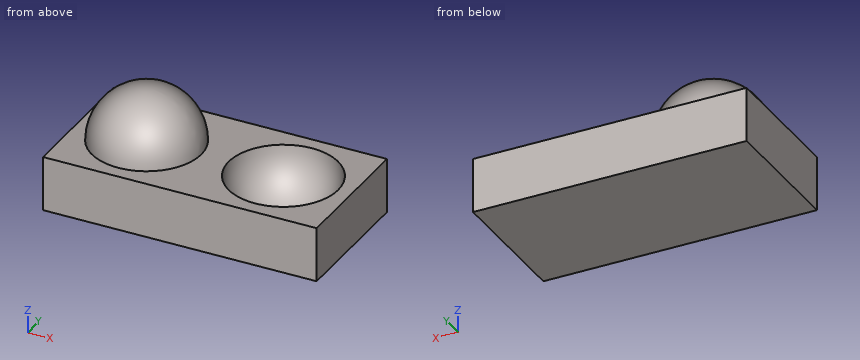
```python
from build123d import *

# Parameters (mm, degrees)
SKETCH_W  = 100
SKETCH_H  = 50
PAD_DEPTH = 20


with BuildPart() as part:
    # Sketch → Pad (new body)
    with BuildSketch(Plane.XY):
        Rectangle(SKETCH_W, SKETCH_H)
    extrude(amount=PAD_DEPTH)

    # Sphere → Sphere (revolve)
    with BuildSketch(Plane(origin=(-25, 0, 20), x_dir=(1, 0, 0), z_dir=(0, -1, 0))):
        with BuildLine():
            ThreePointArc((0, -20), (20, 0), (0, 20))
            Line((0, 20), (0, -20))
        make_face()
    revolve(axis=Axis((-25, 0, 20), (0, 0, 1)))

    # Sphere001 → Sphere001 (revolve, cut)
    with BuildSketch(Plane(origin=(25, 0, 20), x_dir=(1, 0, 0), z_dir=(0, -1, 0))):
        with BuildLine():
            ThreePointArc((0, -20), (20, 0), (0, 20))
            Line((0, 20), (0, -20))
        make_face()
    revolve(axis=Axis((25, 0, 20), (0, 0, 1)), mode=Mode.SUBTRACT)


solid = part.part
```
Input: part model. Units: mm. Frame: model coordinates. Give positions to 0.01 mm unless a question says otherwise; leave off trailing zeros. Write each loop counter-clockwise with the first axis right and the second up, starting at its lowest first coordinate (ties: lowest second). Pieces come first, ordered by that corner, then holes. Notation, with made-up numbers: (-9.75, 9.25) - (17.25, 9.25) arc R30 ccw to (17.25, 36.25) - close; hole circle Ø3 at (-13.75, -37). An arc over 180 degrees is marked (long way). Write item = value, one per line. Start each with the question number.
1) Cut plane A-A (z = 15). Return loops of the section in (x, y).
2) Pin query (flat end, axial travel): pin 1 (2 mm diameter, centred on x = -11.5, z = 30.5, fed in from -Y); pin 2 (1 mm diameter, centred on x = -35, z = 33, fed in from +Y); pin 3 (25 mm diameter, centred on x = -1, y = -2.5, fed in from +Z). Return the tip coordinate at first contact, or that it passes through.
3) Cut plane B-B (x = -9). Return loops of the section in (y, z).
4) Cut plane C-C (y = 15). Return loops of the section in (x, z), and give its area (3 significant figures).
5) Cut plane D-D (z = 31.5). Return loops of the section in (x, y), and give its area (3 significant figures).
6) Material intervals for L1, parallel to X at y = 3, z = 18.5; L2, parallel to X at y = -14.5, z = 15; L3, parallel to Z at x = 10.5, y = 16, sorted ascending. Write a range as [from, to].
Answers follow:
q1.outline = (-50, -25) - (50, -25) - (50, 25) - (-50, 25) - close; hole circle Ø38.73 at (25, 0)
q2.pin_1 = -11.86
q2.pin_2 = 12.13
q2.pin_3 = 36.27
q3.outline = (-25, 0) - (25, 0) - (25, 20) - (12, 20) arc R12 ccw to (-12, 20) - (-25, 20) - close
q4.outline = (-50, 0) - (50, 0) - (50, 20) - (38.23, 20) arc R13.23 cw to (11.77, 20) - (-11.77, 20) arc R13.23 ccw to (-38.23, 20) - (-50, 20) - close
q4.area = 2,000 mm^2
q5.outline = circle Ø32.73 at (-25, 0)
q5.area = 841 mm^2
q6.L1 = [-50, 5.28], [44.72, 50]
q6.L2 = [-50, 12.16], [37.84, 50]
q6.L3 = [0, 20]
